Model file for the job. Use its own axes, mm. Round coordinates to 2 decimals unless told otherwise and drop trailing zeros. Order: outer loops, then holes, each group sorted by start corner. A loop starts at its lowest first (then second) coordinate and runs counter-clockwise, first axis right, second up. Notation, with made-up numbers: (69, -30) -> (87, -30) arc R32 ccw to (87, -4) -> close; hole circle Ø10 at (31.5, 74.25). An arc over 180 degrees is marked (long way). Use CSV: the item, a comma, the result in double quotes.
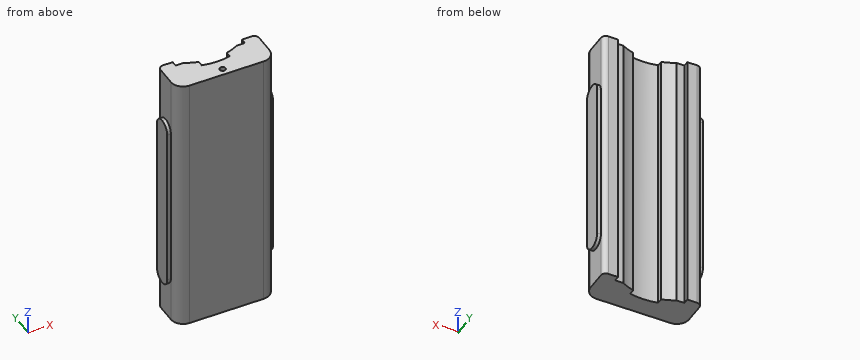
```python
from build123d import *

# Parameters (mm, degrees)
BOSS_EXTRUDE1_DEPTH = 220
FILLET1_R           = 4
FILLET2_R           = 10
SKETCH6_W           = 150
SKETCH6_H           = 16
BOSS_EXTRUDE2_DEPTH = 3
SKETCH7_W           = 150
SKETCH7_H           = 16
BOSS_EXTRUDE3_DEPTH = 3
CUT_EXTRUDE1_DEPTH  = 3
CUT_EXTRUDE2_DEPTH  = 3
SKETCH10_R          = 2.341915658
CUT_EXTRUDE3_DEPTH  = 5
SCALE1_SCALE        = 15.6
SCALE2_SCALE        = 0.5


with BuildPart() as part:
    # Sketch1 → Boss-Extrude1 (new body)
    with BuildSketch(Plane.XY):
        with BuildLine():
            ThreePointArc((39.877280439, -8.639636697), (45.189316192, -6.882935474), (50.242300545, -4.480629882))
            Line((50.242300545, -4.480629882), (56.863188539, -4.480629882))
            Line((56.863188539, -4.480629882), (56.863188539, 0))
            Line((56.863188539, 0), (68.863188539, 0))
            Line((68.863188539, 0), (68.863188539, -30))
            Line((68.863188539, -30), (-12, -30))
            Line((-12, -30), (-12, 0))
            Line((-12, 0), (0, 0))
            Line((0, 0), (0, -4.480629882))
            Line((0, -4.480629882), (6.620887994, -4.480629882))
            ThreePointArc((6.620887994, -4.480629882), (11.673872347, -6.882935474), (16.9859081, -8.639636697))
            Line((16.9859081, -8.639636697), (16.9859081, -13.120266579))
            ThreePointArc((16.9859081, -13.120266579), (28.43159427, -14.466004542), (39.877280439, -13.120266579))
            Line((39.877280439, -13.120266579), (39.877280439, -8.639636697))
        make_face()
    extrude(amount=BOSS_EXTRUDE1_DEPTH)

    # Fillet1
    fillet1_edges = [part.edges().sort_by_distance(p)[0] for p in [
        (68.863188539, 0, 110),
        (-12, 0, 110),
    ]]
    fillet(fillet1_edges, radius=FILLET1_R)

    # Fillet2
    fillet2_edges = [part.edges().sort_by_distance(p)[0] for p in [
        (68.863188539, -30, 110),
        (-12, -30, 110),
    ]]
    fillet(fillet2_edges, radius=FILLET2_R)

    # Sketch6 → Boss-Extrude2 (add)
    with BuildSketch(Plane(origin=(68.863188539, 0, 0), x_dir=(0, 0, -1), z_dir=(1, 0, 0))):
        with Locations((-105, -12)):
            Rectangle(SKETCH6_W, SKETCH6_H)
    extrude(amount=BOSS_EXTRUDE2_DEPTH)

    # Sketch7 → Boss-Extrude3 (add)
    with BuildSketch(Plane.ZY.offset(12)):
        with Locations((104.824258167, -12)):
            Rectangle(SKETCH7_W, SKETCH7_H)
    extrude(amount=BOSS_EXTRUDE3_DEPTH)

    # Sketch8 → Cut-Extrude1 (cut)
    with BuildSketch(Plane.ZY.offset(15)):
        with BuildLine():
            ThreePointArc((37.824258167, -20), (32.167403918, -17.656854249), (29.824258167, -12))
            Line((29.824258167, -12), (29.824258167, -20))
            Line((29.824258167, -20), (37.824258167, -20))
        make_face()
        with BuildLine():
            ThreePointArc((29.824258167, -12), (32.167403918, -6.343145751), (37.824258167, -4))
            Line((37.824258167, -4), (29.824258167, -4))
            Line((29.824258167, -4), (29.824258167, -12))
        make_face()
        with BuildLine():
            Line((179.824258167, -20), (179.824258167, -12))
            ThreePointArc((179.824258167, -12), (177.481112417, -17.656854249), (171.824258167, -20))
            Line((171.824258167, -20), (179.824258167, -20))
        make_face()
        with BuildLine():
            Line((179.824258167, -4), (171.824258167, -4))
            ThreePointArc((171.824258167, -4), (177.481112417, -6.343145751), (179.824258167, -12))
            Line((179.824258167, -12), (179.824258167, -4))
        make_face()
    extrude(amount=-CUT_EXTRUDE1_DEPTH, mode=Mode.SUBTRACT)

    # Sketch9 → Cut-Extrude2 (cut)
    with BuildSketch(Plane(origin=(71.863188539, 0, 0), x_dir=(0, 0, -1), z_dir=(1, 0, 0))):
        with BuildLine():
            ThreePointArc((-180, -12), (-177.656854249, -6.343145751), (-172, -4))
            Line((-172, -4), (-180, -4))
            Line((-180, -4), (-180, -12))
        make_face()
        with BuildLine():
            ThreePointArc((-172, -20), (-177.656854249, -17.656854249), (-180, -12))
            Line((-180, -12), (-180, -20))
            Line((-180, -20), (-172, -20))
        make_face()
        with BuildLine():
            Line((-30, -4), (-38, -4))
            ThreePointArc((-38, -4), (-32.343145751, -6.343145751), (-30, -12))
            Line((-30, -12), (-30, -4))
        make_face()
        with BuildLine():
            Line((-30, -20), (-30, -12))
            ThreePointArc((-30, -12), (-32.343145751, -17.656854249), (-38, -20))
            Line((-38, -20), (-30, -20))
        make_face()
    extrude(amount=-CUT_EXTRUDE2_DEPTH, mode=Mode.SUBTRACT)

    # Sketch10 → Cut-Extrude3 (cut)
    with BuildSketch(Plane.XY.offset(220)):
        with Locations((28.43159427, -23.894216735)):
            Circle(SKETCH10_R)
    extrude(amount=-CUT_EXTRUDE3_DEPTH, mode=Mode.SUBTRACT)


with BuildPart() as part_1:
    # Scale1: scaled about (28.43159427, -17.23906253, 109.80841841)
    add(part.part.scale(SCALE1_SCALE).moved(Location((-415.101276342, 251.690312938, -1603.202908786))))


with BuildPart() as part_2:
    # Scale2: scaled about (28.431594264, -17.23906253, 109.808418405)
    add(part_1.part.scale(SCALE2_SCALE).moved(Location((14.215797132, -8.619531265, 54.904209202))))


solid = part_2.part
```
Q1. Cut at D-D (x = 86.5). Give the cut face in (y, z), plus the area to 3 significant figures.
From the geometry:
outline,"(-116.77, -746.7) -> (8.8, -746.7) -> (8.8, 969.3) -> (-116.77, 969.3) -> close"
area,"215,000 mm²"
Q2. Cut at B-B (x = -116). Give the cut face in (y, z).
From the geometry:
outline,"(-116.77, -746.7) -> (69.39, -746.7) -> (69.39, 969.3) -> (-116.77, 969.3) -> close"
Q3. Cut at A-A (z = 770.5). Give the cut face in (x, y).
From the geometry:
outline,"(-286.93, -38.77) arc R78 ccw to (-208.93, -116.77) -> (265.8, -116.77) arc R78 ccw to (343.8, -38.77) -> (343.8, 86.03) arc R31.2 ccw to (312.6, 117.23) -> (250.2, 117.23) -> (250.2, 82.28) -> (198.56, 82.28) arc R351 cw to (117.71, 49.84) -> (117.71, 14.89) arc R384.9 cw to (-60.84, 14.89) -> (-60.84, 49.84) arc R351 cw to (-141.69, 82.28) -> (-193.33, 82.28) -> (-193.33, 117.23) -> (-255.73, 117.23) arc R31.2 ccw to (-286.93, 86.03) -> close"
Q4. Probe line 1 along X through (y, z) = (22, -151); line 2 along X through (y, z) = (89, -202); line 3 along Y through (x, z) = (-210.5, 884). List the from-to ranges inside material, lowest first.
From the geometry:
line 1,"x = -310.33 to -60.84, 117.71 to 367.2"
line 2,"x = -286.79 to -193.33, 250.2 to 343.66"
line 3,"y = -116.76 to 117.23"
Q5. Pin check, flat tips, straight feed: pin 1 (11.5 mm diameter, centred on x = 359, z = 32.5, fed in from -Y); pin 2 (15.5 mm diameter, centred on x = 215, z = 506, fed in from +Y); pin 3 (10.5 mm diameter, centred on y = 105.5, z = 470.5, fed in from -X). Stop position of each tip, or through.
From the geometry:
pin 1,"stops at y = -38.77"
pin 2,"stops at y = 82.28"
pin 3,"stops at x = -283.5"
Q6. Cut at C-C (z = 6.5). Give the cut face in (x, y).
From the geometry:
outline,"(-310.33, -38.77) -> (-286.93, -38.77) arc R78 ccw to (-208.93, -116.77) -> (265.8, -116.77) arc R78 ccw to (343.8, -38.77) -> (367.2, -38.77) -> (367.2, 86.03) -> (343.8, 86.03) arc R31.2 ccw to (312.6, 117.23) -> (250.2, 117.23) -> (250.2, 82.28) -> (198.56, 82.28) arc R351 cw to (117.71, 49.84) -> (117.71, 14.89) arc R384.9 cw to (-60.84, 14.89) -> (-60.84, 49.84) arc R351 cw to (-141.69, 82.28) -> (-193.33, 82.28) -> (-193.33, 117.23) -> (-255.73, 117.23) arc R31.2 ccw to (-286.93, 86.03) -> (-310.33, 86.03) -> close"
